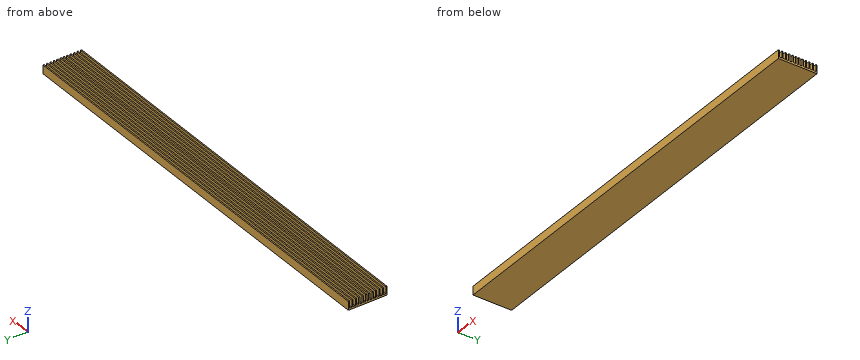
```python
from build123d import *

# Parameters (mm, degrees)
F1_DEPTH = 584.2


with BuildPart() as f1:
    # F0 (on Right) → F1 (new body)
    with BuildSketch(Plane.YZ):
        Polygon((-25.088021, 1.09811), (-26.789821, 1.09811), (-26.789821, -10.68749), (26.016779, -10.68749), (26.016779, 1.09811), (24.314979, 1.09811), (24.314979, -8.19829), (21.317779, -8.19829), (21.317779, 1.09811), (19.615979, 1.09811), (19.615979, -8.19829), (16.618779, -8.19829), (16.618779, 1.09811), (14.916979, 1.09811), (14.916979, -8.19829), (11.919779, -8.19829), (11.919779, 1.09811), (10.217979, 1.09811), (10.217979, -8.19829), (7.220779, -8.19829), (7.220779, 1.09811), (5.518979, 1.09811), (5.518979, -8.19829), (2.521779, -8.19829), (2.521779, 1.09811), (0.819979, 1.09811), (0.819979, -8.19829), (-1.593021, -8.19829), (-1.593021, 1.09811), (-3.294821, 1.09811), (-3.294821, -8.19829), (-6.292021, -8.19829), (-6.292021, 1.09811), (-7.993821, 1.09811), (-7.993821, -8.19829), (-10.991021, -8.19829), (-10.991021, 1.09811), (-12.692821, 1.09811), (-12.692821, -8.19829), (-15.690021, -8.19829), (-15.690021, 1.09811), (-17.391821, 1.09811), (-17.391821, -8.19829), (-20.389021, -8.19829), (-20.389021, 1.09811), (-22.090821, 1.09811), (-22.090821, -8.19829), (-25.088021, -8.19829), align=None)
    extrude(amount=F1_DEPTH)


solid = f1.part
```
Can you work these out from the model? Positions are in its coordinate system, mm. Round coordinates to 2 decimals unless told otherwise and drop trailing zeros.
Item 1: Suppose I cut it at A-A, the plane z = -5.75. State how many separate pieces and enclosed holes the cut face has, then the cut area to 3 significant figures.
Item 2: Please list where this line runs through material, in increasing order: L1, parallel to Z at x = 32, y = -5.
Item 3: Will these pins go through, and if not, where does the flat tip stop? pin 1 Ø1.5 at (x, y) = (180, 8.5) entering from +Z; pin 2 Ø1.5 at (y, z) = (-5.5, -5.5) entering from +X.
Reported:
1. separate pieces: 12
1. enclosed holes: 0
1. area: 11,900 mm2
2. L1: z = -10.69 to -8.2
3. pin 1: stops at z = -8.2
3. pin 2: passes through
